Geometry: final body of the model. Coordinates: model frame, mm. A direction names the side the tool comes from. Give positions to 0.01 mm unless a question says otherwise; leave off trailing zeros. Loops run counter-clockwise (first coordinate to the right, second up) from the corner with the lowest first, then second, coordinate; pieces in that order, holes last. Notation, with made-up numbers: (36.25, -12.75) -> (79.25, -12.75) arc R31 cw to (79.25, 16.25) -> close; hole circle Ø7 at (69.25, -22). An arc over 180 degrees is marked (long way). Answer in a Markdown table with one row per item. Add a question column.
1) Draft query along Y for faces 4 (the cylindrical face through (0, -2, 3)), 5 (the cylindrical face through (-3.25, 0, 2.96)), 6 (the flat face through (0, 4, 0)), 7 (the flat face through (-0.225, -11.4, 2.958)). Return one class per face: +Y half, -Y half, draft (parallel to the pull), parting line (faces both ways), or undercut.
2) Section query B-B (x = 1.5). Give the number of separate pieces and of enclosed holes in the cut face, plus the area to 3 significant figures.
3) Line query: line 1 (X direction, y = -6, z = 3.75); line 2 (Y direction, x = 0, z = 4.2); line 3 (Y direction, x = 0.25, z = 4.5). Output: solid intervals per line, ascending. Write a range as from..to.
4) Access query for faces 1 (the flat face through (1.199, -9, 3)), 2 (the flat face through (0, 4, 6)), 3 (the flat face through (-1.61, -7, 3)). Directions: +Z, -Z, +X, -X, +Y, -Y. A direction counts if a zero-diameter tool reaches every point of the face in a straight line with its end or side. Return the directions, or none.
5) First-contact query: P1, Ø1, axis at x = 1.5, y = 7.5, coming from the -Z side; P2, Ø3, axis at y = 16, z = 1.5, coming from the -X side; P3, Ø3, axis at x = -1.5, z = 1.5, coming from the +Y side; P4, Ø2, axis at y = 16, z = 4.5, coming from the -X side. Flat tips, straight axial feed; report the tip coordinate or a pass-through.
6) Section query A-A (y = -7). Return the cut outline in (x, z).
```python
from build123d import *

# Parameters (mm, degrees)
F0_R     = 2
F1_DEPTH = 6
F2_R     = 2


# Not quite as in the source:
# - a feature names something its author has since deleted; it is built from what else it names


with BuildPart() as f1:
    # F0 (on Top) → F1 (new body)
    with BuildSketch(Plane.XY):
        with BuildLine():
            ThreePointArc((1.1986346156, -3.0208897792), (2.688685785, -1.8257789432), (3.25, 0))
            ThreePointArc((3.25, 0), (2.9473803034, 1.3694704624), (2.0958773247, 2.4839078565))
            ThreePointArc((2.0958773247, 2.4839078565), (0.4368938689, 3.220500543), (-1.3583713088, 2.952512047))
            ThreePointArc((-1.3583713088, 2.952512047), (-3.2469183887, 0.1414955013), (-1.6100655086, -2.8231523264))
            ThreePointArc((-1.6100655086, -2.8231523264), (-0.2282408158, -3.2419756523), (1.1986346156, -3.0208897792))
        make_face()
        Circle(F0_R, mode=Mode.SUBTRACT)
        with BuildLine():
            Line((1.1986346156, -13.0208897792), (1.1986346156, -3.0208897792))
            ThreePointArc((1.1986346156, -3.0208897792), (-0.2282408158, -3.2419756523), (-1.6100655086, -2.8231523264))
            Line((-1.6100655086, -2.8231523264), (-1.6100655086, -9.8231523264))
            Line((-1.6100655086, -9.8231523264), (1.1986346156, -13.0208897792))
        make_face()
        with BuildLine():
            ThreePointArc((-1.3583713088, 2.952512047), (0.4368938689, 3.220500543), (2.0958773247, 2.4839078565))
            ThreePointArc((2.0958773247, 2.4839078565), (0.3587431794, 11.3732693794), (2.2789172363, 20.2248971909))
            add(Edge.make_bspline(
                [(-1.3583713088, 2.952512047), (-3.6481465213, 9.1469325125), (-0.8962951833, 19.0959330648), (2.2789172363, 20.2248971909)],
                knots=[0, 0, 0, 0, 17.6512083587, 17.6512083587, 17.6512083587, 17.6512083587], degree=3))
        make_face()
    extrude(amount=F1_DEPTH)

    # F2
    f2_edges = [f1.edges().sort_by_distance(p)[0] for p in [
        (-1.610066, -2.823152, 3),
        (1.198635, -3.02089, 3),
        (-1.358371, 2.952512, 3),
        (2.095877, 2.483908, 3),
    ]]
    fillet(f2_edges, radius=F2_R)


solid = f1.part
```
Evaluation:
| question | item | result |
|---|---|---|
| 1 | face 4 | undercut |
| 1 | face 5 | parting line |
| 1 | face 6 | draft |
| 1 | face 7 | -Y half |
| 2 | separate pieces | 3 |
| 2 | enclosed holes | 0 |
| 2 | area | 36.6 mm² |
| 3 | line 1 | -1.61..1.2 |
| 3 | line 2 | -11.66..-2, 2..17.83 |
| 3 | line 3 | -11.94..-1.98, 1.98..18.26 |
| 4 | face 1 | +Z, -Z, +X, -Y |
| 4 | face 2 | +Z, +X, -X, +Y, -Y |
| 4 | face 3 | +Z, -Z, -X, -Y |
| 5 | P1 | through |
| 5 | P2 | x = -1.33 |
| 5 | P3 | y = 17.83 |
| 5 | P4 | x = -1.18 |
| 6 | outline | (-1.61, 0) -> (1.2, 0) -> (1.2, 6) -> (-1.61, 6) -> close |
